Can you work these out from the drawing? Everything is in mm from the part's minimum corner. A direction names the side the tool comes from. Coordinates: 2 decimals unless noted, no trailing zeros. Loops run counter-clockwise (first coordinate to the right, second up) from the corner with the lowest first, then second, coordinate; pieces in that order, holes last. Notation, with made-up numbers: M 84,-3 L 113,-3 A24 ccw 113,22 Z; hole C -9.75,7.25 d6. An arc over 180 degrees is marked long. Write each question's results on one line, items separated by ' | '.
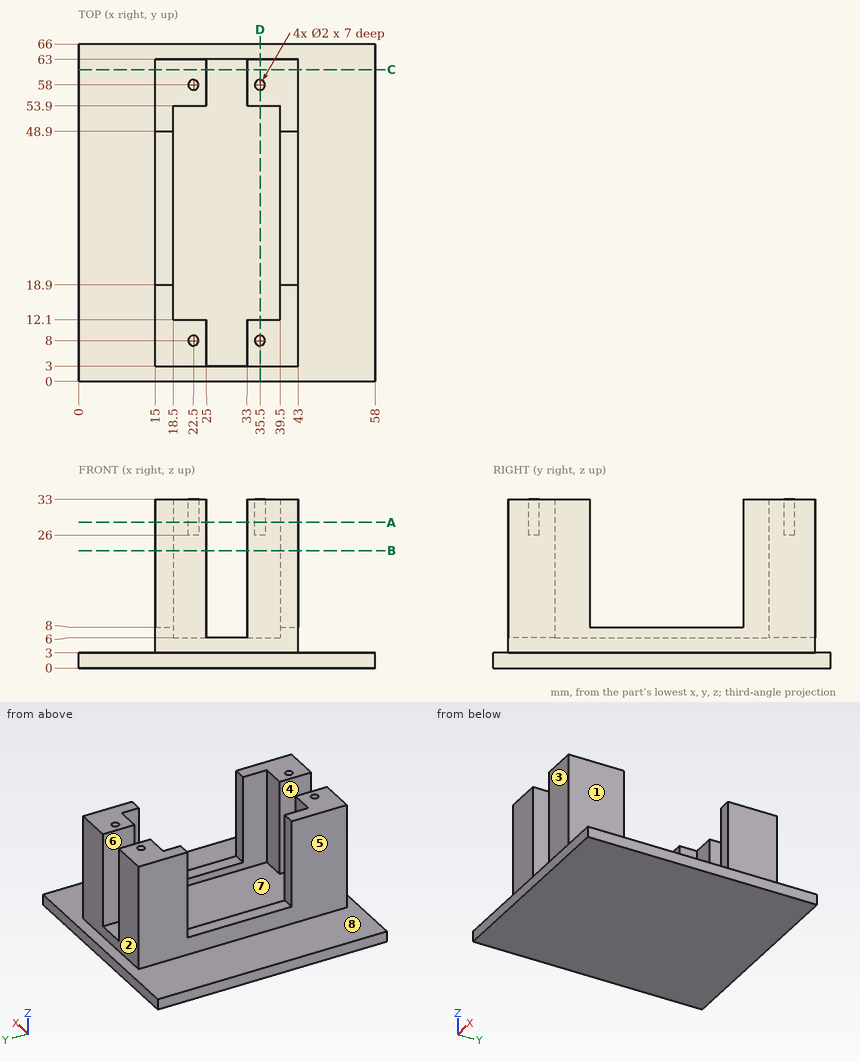
(1) Imagine slicing it at A-A, the plane z = 28.5. List the corners of the cut face in (x, y) for me, and give its area (3 significant figures).
Reported:
outline: M 15,3 L 25,3 L 25,12.1 L 18.5,12.1 L 18.5,18.9 L 15,18.9 Z; M 15,48.9 L 18.5,48.9 L 18.5,53.9 L 25,53.9 L 25,63 L 15,63 Z; M 33,3 L 43,3 L 43,18.9 L 39.5,18.9 L 39.5,12.1 L 33,12.1 Z; M 33,53.9 L 39.5,53.9 L 39.5,48.9 L 43,48.9 L 43,63 L 33,63 Z; hole C 22.5,8 d2; hole C 22.5,58 d2; hole C 35.5,8 d2; hole C 35.5,58 d2 | area: 434 mm2
(2) Which directions (+Z, -Z, +X, -X, +Y, -Y) give clear straight access to the entire face, cutting with the end or side of a thin tool? Please do the marked faces 1, 2, 3 and 4.
Reported:
face 1: +Z, +X, +Y, -Y | face 2: +Z, +X, -X, +Y | face 3: +Z, +X, -X, -Y | face 4: +Z, +Y, -Y
(3) Imagine slicing it at D-D, the plane x = 35.5. List the corners of the cut face in (y, z) for me, and give its area (3 significant figures).
Reported:
outline: M 0,0 L 66,0 L 66,3 L 63,3 L 63,33 L 59,33 L 59,26 L 57,26 L 57,33 L 53.9,33 L 53.9,6 L 12.1,6 L 12.1,33 L 9,33 L 9,26 L 7,26 L 7,33 L 3,33 L 3,3 L 0,3 Z | area: 841 mm2
(4) Imagine slicing it at C-C, the plane y = 61. List the corners of the cut face in (x, z) for me, and give its area (3 significant figures).
Reported:
outline: M 0,0 L 58,0 L 58,3 L 43,3 L 43,33 L 33,33 L 33,6 L 25,6 L 25,33 L 15,33 L 15,3 L 0,3 Z | area: 798 mm2
(5) Please list where these lines run through material, in increasing order: probe 1 along X at (y, z) = (58, 29); probe 2 along Y at (x, z) = (22.5, 27.5); probe 3 along Y at (x, z) = (21.5, 17.5). Write a range as from..to.
Reported:
probe 1: x = 15..21.5, 23.5..25, 33..34.5, 36.5..43 | probe 2: y = 3..7, 9..12.1, 53.9..57, 59..63 | probe 3: y = 3..12.1, 53.9..63
(6) Will these pins go through, and if not, where does the flat tip stop? P1, Ø4.5, axis at y = 8.5, z = 17.5, coming from the +X side; P2, Ø1.5, axis at x = 23, y = 28, coming from the -Z side; P3, Ø1, axis at x = 41, z = 21, coming from the +Y side; P4, Ø9, axis at y = 42, z = 11, coming from the -X side.
Reported:
P1: stops at x = 43 | P2: stops at z = 0 | P3: stops at y = 63 | P4: stops at x = 15
(7) If we mould it in two halves opening along X, with no side actions, what happens to the marked faces 5, 6, 7 and 8? For each: released by +X, released by -X, zero draft, split by the parting line, or undercut.
Reported:
face 5: released by -X | face 6: undercut | face 7: undercut | face 8: zero draft
(8) Imagine slicing it at B-B, the plane z = 23. List the corners of the cut face in (x, y) for me.
Reported:
outline: M 15,3 L 25,3 L 25,12.1 L 18.5,12.1 L 18.5,18.9 L 15,18.9 Z; M 15,48.9 L 18.5,48.9 L 18.5,53.9 L 25,53.9 L 25,63 L 15,63 Z; M 33,3 L 43,3 L 43,18.9 L 39.5,18.9 L 39.5,12.1 L 33,12.1 Z; M 33,53.9 L 39.5,53.9 L 39.5,48.9 L 43,48.9 L 43,63 L 33,63 Z
